```python
from build123d import *

# Parameters (mm, degrees)
F1_DEPTH = 38.1
F2_R     = 30.48
F3_DEPTH = 38.1
F4_R     = 30.48


with BuildPart() as f1:
    # F0 (on Top) → F1 (new body)
    with BuildSketch(Plane.XY):
        with BuildLine():
            Line((-139.7, -152.4), (139.7, -152.4))
            ThreePointArc((139.7, -152.4), (175.6210244843, -137.5210244843), (190.5, -101.6))
            Line((190.5, -101.6), (190.5, 101.6))
            ThreePointArc((190.5, 101.6), (175.6210244843, 137.5210244843), (139.7, 152.4))
            Line((139.7, 152.4), (-139.7, 152.4))
            ThreePointArc((-139.7, 152.4), (-175.6210244843, 137.5210244843), (-190.5, 101.6))
            Line((-190.5, 101.6), (-190.5, -101.6))
            ThreePointArc((-190.5, -101.6), (-175.6210244843, -137.5210244843), (-139.7, -152.4))
        make_face()
    extrude(amount=F1_DEPTH)

    # F2
    f2_edges = [f1.edges().sort_by_distance(p)[0] for p in [
        (0, -152.4, 0),
    ]]
    fillet(f2_edges, radius=F2_R)

    # F3 (add): a face of the model
    f3_faces = [f1.faces().sort_by_distance(p)[0] for p in [
        (0, 0, 38.1),
    ]]
    extrude(f3_faces, amount=F3_DEPTH)

    # F4
    f4_edges = [f1.edges().sort_by_distance(p)[0] for p in [
        (0, -152.4, 76.2),
    ]]
    fillet(f4_edges, radius=F4_R)


solid = f1.part
```
The listing builds one solid part. Answer for the finished solid, in the listing's coordinates (mm). Give positions to 0.01 mm unless a question says otherwise; leave off trailing zeros. Order: outer loops, then holes, each group sorted by start corner. A loop starts at its lowest first (then second) coordinate and runs counter-clockwise, first axis right, second up. Notation, with made-up numbers: (30.5, 30) -> (89.5, 30) arc R14 cw to (89.5, 56) -> close; hole circle Ø8 at (51, 67). An arc over 180 degrees is marked (long way). Write each question's results on one line, items separated by ' | '.
Q1. The part is cut by section A-A, the plane y = -73.5. Give the vertices of the cut face in (x, z), and give its area (3 significant figures).
Checked values:
outline: (-190.5, 30.48) arc R30.48 ccw to (-160.02, 0) -> (160.02, 0) arc R30.48 ccw to (190.5, 30.48) -> (190.5, 45.72) arc R30.48 ccw to (160.02, 76.2) -> (-160.02, 76.2) arc R30.48 ccw to (-190.5, 45.72) -> close | area: 28,200 mm^2
Q2. The part is cut by section B-B, the plane z = 37.5. Give the vertices of the cut face in (x, y), and give its area (3 significant figures).
Checked values:
outline: (-190.5, -101.6) arc R50.8 ccw to (-139.7, -152.4) -> (139.7, -152.4) arc R50.8 ccw to (190.5, -101.6) -> (190.5, 101.6) arc R50.8 ccw to (139.7, 152.4) -> (-139.7, 152.4) arc R50.8 ccw to (-190.5, 101.6) -> close | area: 114,000 mm^2
Q3. Straight lines are drawn through the part: probe 1 along Y at (x, z) = (96.5, 19.5); probe 2 along Y at (x, z) = (-60, 64); probe 3 along X at (y, z) = (-3, 10). For each, find the intervals that lie inside material, in ascending order. Write a range as from..to.
Checked values:
probe 1: y = -150.35..150.35 | probe 2: y = -146.31..146.31 | probe 3: x = -182.59..182.59
Q4. Each of these flat-tipped pins is pushed along its axis until it touches: P1, Ø2, axis at y = 37.5, z = 62, coming from the +X side; P2, Ø2, axis at x = -16, z = 21, coming from the +Y side; P3, Ø2, axis at y = 78, z = 19.5, coming from the -X side. Where does it stop, or does it pass through?
Checked values:
P1: stops at x = 186.39 | P2: stops at y = 151.2 | P3: stops at x = -188.82
